```python
from build123d import *

# Parameters (mm, degrees)
BOSS_EXTRUDE1_DEPTH = 12
BOSS_EXTRUDE2_DEPTH = 2
CUT_EXTRUDE1_DEPTH  = 3
FILLET1_R           = 3
FILLET2_R           = 3
HOLE2_D             = 10
HOLE3_D             = 10
HOLE4_D             = 10
HOLE5_D             = 10


with BuildPart() as part:
    # Sketch1 → Boss-Extrude1 (new body)
    with BuildSketch(Plane(origin=(0, 0, 0), x_dir=(1, 0, 0), z_dir=(0, 1, 0))):
        with BuildLine():
            Line((-76.865222767, 28.026373193), (57.134777233, 28.026373193))
            ThreePointArc((57.134777233, 28.026373193), (65.620058607, 24.511654567), (69.134777233, 16.026373193))
            Line((69.134777233, 16.026373193), (69.134777233, -33.973626807))
            ThreePointArc((69.134777233, -33.973626807), (65.620058607, -42.458908182), (57.134777233, -45.973626807))
            Line((57.134777233, -45.973626807), (-76.865222767, -45.973626807))
            ThreePointArc((-76.865222767, -45.973626807), (-85.350504141, -42.458908182), (-88.865222767, -33.973626807))
            Line((-88.865222767, -33.973626807), (-88.865222767, 16.026373193))
            ThreePointArc((-88.865222767, 16.026373193), (-85.350504141, 24.511654567), (-76.865222767, 28.026373193))
        make_face()
    extrude(amount=BOSS_EXTRUDE1_DEPTH)

    # Sketch2 → Boss-Extrude2 (add)
    with BuildSketch(Plane(origin=(0, 12, 0), x_dir=(-1, 0, 0), z_dir=(0, 1, 0))):
        Polygon((9.865222767, -28.026373193), (42.865222767, -28.026373193), (42.865222767, 45.973626807), (-23.134777233, 45.973626807), (-23.134777233, -28.026373193), align=None)
    extrude(amount=BOSS_EXTRUDE2_DEPTH)

    # Sketch3 → Cut-Extrude1 (cut)
    with BuildSketch(Plane.XZ):
        Polygon((-9.865222767, 45.973626807), (19.134777233, 45.973626807), (19.134777233, -28.026373193), (-38.865222767, -28.026373193), (-38.865222767, 45.973626807), align=None)
    extrude(amount=-CUT_EXTRUDE1_DEPTH, mode=Mode.SUBTRACT)

    # Fillet1
    fillet1_edges = [part.edges().sort_by_distance(p)[0] for p in [
        (-38.865222767, 3, 8.973626807),
    ]]
    fillet(fillet1_edges, radius=FILLET1_R - 0.0001)  # a hair under: the kernel refuses the full size

    # Fillet2
    fillet2_edges = [part.edges().sort_by_distance(p)[0] for p in [
        (19.134777233, 3, 8.973626807),
    ]]
    fillet(fillet2_edges, radius=FILLET2_R - 0.0001)  # a hair under: the kernel refuses the full size

    # Hole2 (through all)
    with Locations(Plane(origin=(0, 12, 0), x_dir=(-1, 0, 0), z_dir=(0, 1, 0))):
        with Locations((76.865222767, -16.026373193)):
            Hole(HOLE2_D / 2)

    # Hole3 (through all)
    with Locations(Plane(origin=(0, 12, 0), x_dir=(-1, 0, 0), z_dir=(0, 1, 0))):
        with Locations((76.865222767, 33.973626807)):
            Hole(HOLE3_D / 2)

    # Hole4 (through all)
    with Locations(Plane(origin=(0, 12, 0), x_dir=(-1, 0, 0), z_dir=(0, 1, 0))):
        with Locations((-57.134777233, 33.973626807)):
            Hole(HOLE4_D / 2)

    # Hole5 (through all)
    with Locations(Plane(origin=(0, 12, 0), x_dir=(-1, 0, 0), z_dir=(0, 1, 0))):
        with Locations((-57.134777233, -16.026373193)):
            Hole(HOLE5_D / 2)


solid = part.part
```
Could you check a few things on this model? Use its own coordinates, in mm. A direction names the side the tool comes from. Round coordinates to 2 decimals unless told otherwise and drop trailing zeros. Loops run counter-clockwise (first coordinate to the right, second up) from the corner with the lowest first, then second, coordinate; pieces in that order, holes last. Notation, with made-up numbers: (18.25, -17) -> (29.25, -17) arc R18 cw to (29.25, -13) -> close; hole circle Ø3 at (61.5, 20). An arc over 180 degrees is marked (long way). One line per question, with ' | ' between items.
(1) For pin 1 Ø1.6 at (y, z) = (13.5, 2.5) entering from -X; pin 2 Ø13 at (x, z) = (-76.87, -16.03) entering from +Y; pin 3 Ø10 at (x, z) = (-25.5, 19) entering from -Y, each with a flat end and sliding along its axis, tell me the tip position at first contact or that it passes through.
Model answer:
pin 1: stops at x = -42.87 | pin 2: stops at y = 12 | pin 3: stops at y = 3
(2) Thinking about a two-plate mould opening in X: for faces 1 (the face through (-88.865, 6, 9)), 2 (the face through (-38.01, 2.1, 9.49)), 3 (the face through (65.53, 5.92, -24.6)), 4 (the face through (-11, 7, -28.026)), which applies, released by +X, released by -X, zero draft, split by the parting line, or undercut?
Model answer:
face 1: released by -X | face 2: undercut | face 3: released by +X | face 4: zero draft
(3) If we section it at C-C on x = -57: List the corners of the cut face in (y, z) for me.
Model answer:
outline: (0, -28.03) -> (12, -28.03) -> (12, 45.97) -> (0, 45.97) -> close
(4) If we section it at A-A on y = 7.25: List the corners of the cut face in (x, z) for me.
Model answer:
outline: (-88.87, -16.03) arc R12 ccw to (-76.87, -28.03) -> (57.13, -28.03) arc R12 ccw to (69.13, -16.03) -> (69.13, 33.97) arc R12 ccw to (57.13, 45.97) -> (-76.87, 45.97) arc R12 ccw to (-88.87, 33.97) -> close; hole circle Ø10 at (-76.87, -16.03); hole circle Ø10 at (-76.87, 33.97); hole circle Ø10 at (57.13, -16.03); hole circle Ø10 at (57.13, 33.97)
(5) For faces 5 (the face through (-66, 12, 8)), 6 (the face through (46, 12, 8)), 7 (the face through (18.233, 2.145, 8.456)), which set-ups out of +Z, -Z, +X, -X, +Y, -Y let a thin tool reach every point of the face, with its end or its side?
Model answer:
face 5: +Z, -Z, -X, +Y | face 6: +Z, -Z, +X, +Y | face 7: +Z, -Z, -Y
(6) If I drill on probe 1 along Z at (x, y) = (-79.5, 5); probe 2 along Y at (x, z) = (-50, -21.5); probe 3 along X at (y, z) = (13.25, 16.5), over which ranges is the centre line in solid material (lowest first)?
Model answer:
probe 1: z = -27.73 to -20.28, -11.78 to 29.72, 38.22 to 45.68 | probe 2: y = 0 to 12 | probe 3: x = -42.87 to 23.13
